CAD build for the part. Positions are in the model's coordinates, mm. A direction names the side the tool comes from. Coordinates: 2 decimals unless noted, no trailing zeros. Order: outer loops, then holes, each group sorted by start corner. A loop starts at its lowest first (then second) coordinate and runs counter-clockwise, first axis right, second up.
Autodesk Inventor part; units mm, degrees
ref_plane "YZ Plane" through (0, 0, 0) normal (1, 0, 0) x (0, 1, 0)
ref_plane "XZ Plane" through (0, 0, 0) normal (0, 1, 0) x (-1, 0, 0)
ref_plane "XY Plane" through (0, 0, 0) normal (0, 0, 1) x (1, 0, 0)
sketch "Sketch1" plane through (0, 0, 0) normal (0, 0, 1) x (1, 0, 0)
  line L0 (-2.5, -18) -> (2.5, -18)
  line L1 (2.5, -18) -> (2.5, 18)
  line L2 (2.5, 18) -> (-2.5, 18)
  line L3 (-2.5, 18) -> (-2.5, -18)
  line L4 (-2.5, -18) -> (2.5, 18) construction
  line L5 (2.5, -18) -> (-2.5, 18) construction
  line L6 (2.5, 0) -> (20.5, 18)
  line L7 (20.5, 18) -> (2.5, 18)
  line L8 (-7.1, 0) -> (25.1, 0)
  line L9 (2.5, 0) -> (20.5, -18)
  line L10 (20.5, -18) -> (2.5, -18)
  line L11 (15.5, 18) -> (15.5, 13)
  line L12 (15.5, -18) -> (15.5, -13)
  line L13 (7.5, 5) -> (7.5, -5)
  point P0 (0, 0)
  point P1 (15.5, -13)
  dimension "d1" = 5
  dimension "d3" = 45
  dimension "d4" = 18
  dimension "d5" = 5
  dimension "d6" = 5
extrude "Extrusion1" add sketch "Sketch1" along normal blind 10 contours L3 L8 L1 L0 | L1 L9 L12 L10 | L3 L2 L1 L8 | L1 L7 L11 L6 | L6 L13 L8 | L8 L13 L9
properties part number "_3DPrint"
1) Slice it at C-C (y = 0). List the corners of the cut face in (x, z).
2) Which spindle directions (+Z, -Z, +X, -X, +Y, -Y) get a long thin tool onto all of the face, cutting with end or side? Do faces 1 (the flat face through (15.5, 16, 5)), 2 (the flat face through (7.5, 0, 5)). Say none if no direction does.
3) Drill centre lines: probe 1 along X at (y, z) = (3.5, 6.5); probe 2 along Y at (x, z) = (13, 3.75); probe 3 along Y at (x, z) = (8, 5.5). Where is each one in solid material? Low to high.
4) Slice it at A-A (x = 8.75). List the corners of the cut face in (y, z).
5) Slice it at B-B (z = 3.5). List the corners of the cut face in (x, y), plus the area to 3 significant figures.
6) Slice it at D-D (x = 13.5). List the corners of the cut face in (y, z).
Worked out:
1. outline: (-2.5, 0) - (7.5, 0) - (7.5, 10) - (-2.5, 10) - close
2. face 1: +Z, -Z, +X, +Y, -Y
2. face 2: +Z, -Z, +X
3. probe 1: x = -2.5 to 7.5
3. probe 2: y = -18 to -10.5, 10.5 to 18
3. probe 3: y = -18 to -5.5, 5.5 to 18
4. outline: (-18, 0) - (-6.25, 0) - (-6.25, 10) - (-18, 10) - close; (6.25, 0) - (18, 0) - (18, 10) - (6.25, 10) - close
5. outline: (-2.5, -18) - (15.5, -18) - (15.5, -13) - (7.5, -5) - (7.5, 5) - (15.5, 13) - (15.5, 18) - (-2.5, 18) - close
5. area: 504 mm2
6. outline: (-18, 0) - (-11, 0) - (-11, 10) - (-18, 10) - close; (11, 0) - (18, 0) - (18, 10) - (11, 10) - close
